Read the model definition and answer for the solid it produces. Units are mm, in the model's axes. A direction names the side the tool comes from. Round coordinates to 2 decimals unless told otherwise and drop trailing zeros. Order: outer loops, then holes, each group sorted by start corner. A loop starts at its lowest first (then second) coordinate and runs counter-clockwise, first axis right, second up. Notation, with made-up numbers: (19.25, -39) - (38.25, -39) arc R24 cw to (38.25, -13) - close; hole circle Ø4 at (3, -30.75). An arc over 180 degrees is marked (long way). Put each result on its own line as item: value. Start each with the question number.
Q1. Section C-C on z = 0 is taken. Give the vertices of the cut face in (x, y) (3 decimals), then the cut area to 3 significant figures.
Q2. Each of these flat-tipped pins is pushed along its axis until it touches: pin 1 Ø1.2 at (x, y) = (11, -14.5) entering from +Z; pin 2 Ø8 at (x, y) = (16, -9) entering from -Z; pin 3 Ø6 at (x, z) = (-22, -4) entering from +Y. Where does it stop, or does it pass through?
Q3. Section A-A on x = 0 is taken. Give the vertices of the cut face in (y, z) (3 decimals), then the cut area to 3 significant figures.
Q4. For a pull along Y with two mould halves and no side action, classify faces 1 (the face through (-1, -15.875, 19)), 2 (the face through (42, -11, 42.5)), 3 (the face through (44, 0, 1)), 4 (the face through (-45, -11, -32.5)) as pulls with the +Y half, pulls with the -Y half, needs draft (parallel to the pull), parting line crosses it, or undercut.
Q5. Find the intervals of material crossed by line 1 along Z through (x, y) = (-16.5, -13); line 2 along X through (y, z) = (-7, -16.5); line 3 along X through (y, z) = (-5, 19), in increasing order. Write a range as from..to.
Q6. Section B-B on y = -1.75 is taken. Give the vertices of the cut face in (x, z).
Q7. Which of the six approach directions +Z, -Z, +X, -X, +Y, -Y give full straight-line access (tool end or side, diameter ignored) to faces 5 (the face through (39.25, -11, -41)), 6 (the face through (-1, -14, 34.5)), 7 (the face through (-45, -11, 37.5)), 8 (the face through (43.896, -2.896, 35.545))?
Q8. Section D-D on x = -34.75 is taken. Give the vertices of the cut face in (y, z) (3 decimals).
from build123d import *

# Parameters (mm, degrees)
F0_W      = 101.5
F0_H      = 85
F1_DEPTH  = 15.875
F2_R      = 16.25
F3_DEPTH  = 25
F4_W      = 101.5
F4_H      = 85
F5_DEPTH  = 5.875
F7_DEPTH  = 12
F8_W      = 78.5
F8_H      = 10
F9_DEPTH  = 3.5
F10_W     = 78.5
F10_H     = 10
F11_DEPTH = 3.5
F12_W     = 78.5
F12_H     = 3
F13_DEPTH = 25
F14_W     = 78.5
F14_H     = 17.569206
F15_DEPTH = 200
F16_W     = 78.5
F16_H     = 75
F17_DEPTH = 6.125
F18_R     = 1.5
F18_W     = 66.5
F18_H     = 3
F19_DEPTH = 2
F20_R     = 1.5
F20_W     = 66.5
F20_H     = 3
F21_DEPTH = 2
F22_R     = 2.5
F23_DEPTH = 10
F24_R     = 2.5
F25_DEPTH = 10
F26_R     = 2.5
F27_DEPTH = 5
F28_R     = 2.5
F29_DEPTH = 5


with BuildPart() as f1:
    # F0 (on Front) → F1 (new body)
    with BuildSketch(Plane.XZ):
        Rectangle(F0_W, F0_H)
    extrude(amount=F1_DEPTH)

    # F2 (on face) → F3 (cut)
    with BuildSketch(Plane.XZ.offset(15.875)):
        Circle(F2_R)
    extrude(amount=-F3_DEPTH, mode=Mode.SUBTRACT)

    # F4 (on face) → F5 (cut)
    with BuildSketch(Plane(origin=(0, 0, 0), x_dir=(-1, 0, 0), z_dir=(0, 1, 0))):
        Rectangle(F4_W, F4_H)
        with BuildLine():
            Line((-45.75, -31), (-45.75, 31))
            ThreePointArc((-45.75, 31), (-43.846194, 35.596194), (-39.25, 37.5))
            Line((-39.25, 37.5), (39.25, 37.5))
            ThreePointArc((39.25, 37.5), (43.846194, 35.596194), (45.75, 31))
            Line((45.75, 31), (45.75, -31))
            ThreePointArc((45.75, -31), (43.846194, -35.596194), (39.25, -37.5))
            Line((39.25, -37.5), (-39.25, -37.5))
            ThreePointArc((-39.25, -37.5), (-43.846194, -35.596194), (-45.75, -31))
        make_face(mode=Mode.SUBTRACT)
    extrude(amount=-F5_DEPTH, mode=Mode.SUBTRACT)

    # F6 (on face) → F7 (cut)
    with BuildSketch(Plane(origin=(0, 0, 0), x_dir=(-1, 0, 0), z_dir=(0, 1, 0))):
        with BuildLine():
            ThreePointArc((-36.25, 34.5), (-40.846194, 32.596194), (-42.75, 28))
            Line((-42.75, 28), (-42.75, -28))
            ThreePointArc((-42.75, -28), (-40.846194, -32.596194), (-36.25, -34.5))
            Line((-36.25, -34.5), (36.25, -34.5))
            ThreePointArc((36.25, -34.5), (40.846194, -32.596194), (42.75, -28))
            Line((42.75, -28), (42.75, 28))
            ThreePointArc((42.75, 28), (40.846194, 32.596194), (36.25, 34.5))
            Line((36.25, 34.5), (-36.25, 34.5))
        make_face()
    extrude(amount=-F7_DEPTH, mode=Mode.SUBTRACT)

    # F8 (on face) → F9 (cut)
    with BuildSketch(Plane.XY.offset(42.5)):
        with Locations((0, -10.875)):
            Rectangle(F8_W, F8_H)
    extrude(amount=-F9_DEPTH, mode=Mode.SUBTRACT)

    # F10 (on face) → F11 (cut)
    with BuildSketch(Plane(origin=(0, 0, -42.5), x_dir=(1, 0, 0), z_dir=(0, 0, -1))):
        with Locations((0, 10.875)):
            Rectangle(F10_W, F10_H)
    extrude(amount=-F11_DEPTH, mode=Mode.SUBTRACT)

    # F12 (on face) → F13 (cut)
    with BuildSketch(Plane.XZ.offset(15.875)):
        with Locations((0, 36)):
            Rectangle(F12_W, F12_H)
        with Locations((0, -36)):
            Rectangle(F12_W, F12_H)
    extrude(amount=-F13_DEPTH, mode=Mode.SUBTRACT)

    # F14 (on face) → F15 (cut)
    with BuildSketch(Plane.XY.offset(39)):
        with Locations((0, 2.909603)):
            Rectangle(F14_W, F14_H)
    extrude(amount=-F15_DEPTH, mode=Mode.SUBTRACT)

    # F16 (on face) → F17 (cut)
    with BuildSketch(Plane(origin=(0, -5.875, 0), x_dir=(-1, 0, 0), z_dir=(0, 1, 0))):
        Rectangle(F16_W, F16_H)
    extrude(amount=-F17_DEPTH, mode=Mode.SUBTRACT)

    # F18 (on face) → F19 (cut)
    with BuildSketch(Plane.XY.offset(39)):
        with Locations((-34.75, -10.375)):
            Circle(F18_R)
        with Locations((3, -10.375)):
            Rectangle(F18_W, F18_H)
    extrude(amount=-F19_DEPTH, mode=Mode.SUBTRACT)

    # F20 (on face) → F21 (cut)
    with BuildSketch(Plane(origin=(0, 0, -39), x_dir=(1, 0, 0), z_dir=(0, 0, -1))):
        with Locations((34.75, 10.375)):
            Circle(F20_R)
        with Locations((-3, 10.375)):
            Rectangle(F20_W, F20_H)
    extrude(amount=-F21_DEPTH, mode=Mode.SUBTRACT)

    # F22 (on face) → F23 (cut)
    with BuildSketch(Plane(origin=(0, 0, -42.5), x_dir=(1, 0, 0), z_dir=(0, 0, -1))):
        with Locations((-45, 10.875)):
            Circle(F22_R)
    extrude(amount=-F23_DEPTH, mode=Mode.SUBTRACT)

    # F24 (on face) → F25 (cut)
    with BuildSketch(Plane(origin=(0, 0, -42.5), x_dir=(1, 0, 0), z_dir=(0, 0, -1))):
        with Locations((45, 10.875)):
            Circle(F24_R)
    extrude(amount=-F25_DEPTH, mode=Mode.SUBTRACT)

    # F26 (on face) → F27 (cut)
    with BuildSketch(Plane.XY.offset(42.5)):
        with Locations((-45, -10.875)):
            Circle(F26_R)
    extrude(amount=-F27_DEPTH, mode=Mode.SUBTRACT)

    # F28 (on face) → F29 (cut)
    with BuildSketch(Plane.XY.offset(42.5)):
        with Locations((45, -10.875)):
            Circle(F28_R)
    extrude(amount=-F29_DEPTH, mode=Mode.SUBTRACT)


solid = f1.part
Findings:
1. outline: (-50.75, -15.875) - (-16.25, -15.875) - (-16.25, -12) - (-42.75, -12) - (-42.75, 0) - (-45.75, 0) - (-45.75, -5.875) - (-50.75, -5.875) - close; (16.25, -15.875) - (50.75, -15.875) - (50.75, -5.875) - (45.75, -5.875) - (45.75, 0) - (42.75, 0) - (42.75, -12) - (16.25, -12) - close
1. area: 401 mm2
2. pin 1: z = 39
2. pin 2: z = -39
2. pin 3: y = -12
3. outline: (-15.875, -39) - (-11.875, -39) - (-11.875, -37.5) - (-15.875, -37.5) - close; (-15.875, -34.5) - (-12, -34.5) - (-12, -16.25) - (-15.875, -16.25) - close; (-15.875, 16.25) - (-12, 16.25) - (-12, 34.5) - (-15.875, 34.5) - close; (-15.875, 37.5) - (-11.875, 37.5) - (-11.875, 39) - (-15.875, 39) - close; (-8.875, -39) - (-5.875, -39) - (-5.875, -37.5) - (-8.875, -37.5) - close; (-8.875, 37.5) - (-5.875, 37.5) - (-5.875, 39) - (-8.875, 39) - close
3. area: 162 mm2
4. face 1: pulls with the -Y half
4. face 2: needs draft
4. face 3: pulls with the +Y half
4. face 4: undercut
5. line 1: -39..-37.5, -34.5..34.5, 37.5..39
5. line 2: -50.75..-42.75, 42.75..50.75
5. line 3: -45.75..-42.75, 42.75..45.75
6. outline: (-45.75, -31) arc R6.5 ccw to (-39.25, -37.5) - (-39.25, -33.77) arc R6.5 cw to (-42.75, -28) - (-42.75, 28) arc R6.5 cw to (-39.25, 33.77) - (-39.25, 37.5) arc R6.5 ccw to (-45.75, 31) - close; (39.25, -37.5) arc R6.5 ccw to (45.75, -31) - (45.75, 31) arc R6.5 ccw to (39.25, 37.5) - (39.25, 33.77) arc R6.5 cw to (42.75, 28) - (42.75, -28) arc R6.5 cw to (39.25, -33.77) - close
7. face 5: -Z, +Y, -Y
7. face 6: +Y, -Y
7. face 7: +Z
7. face 8: +Z, +X, +Y
8. outline: (-15.875, -39) - (-11.875, -39) - (-11.875, -37.5) - (-15.875, -37.5) - close; (-15.875, -34.5) - (-12, -34.5) - (-12, 34.5) - (-15.875, 34.5) - close; (-15.875, 37.5) - (-11.875, 37.5) - (-11.875, 39) - (-15.875, 39) - close; (-8.875, -39) - (-5.875, -39) - (-5.875, -37.5) - (-8.875, -37.5) - close; (-8.875, 37.5) - (-5.875, 37.5) - (-5.875, 39) - (-8.875, 39) - close
